from build123d import *

# Parameters (mm, degrees)
F1_DEPTH = 24
F3_DEPTH = 13


with BuildPart() as f1:
    # F0 (on Front) → F1 (new body)
    with BuildSketch(Plane.XZ):
        Polygon((30.517951, 0), (-33.758782, 0), (-56.984834, -93.20651), (58.065102, -93.20651), align=None)
    extrude(amount=F1_DEPTH)

    # F2 (on face) → F3 (join)
    with BuildSketch(Plane.XZ.offset(24)):
        Polygon((-51.863408, -72.654148), (-56.984834, -93.20651), (58.065102, -93.20651), (51.990858, -72.654148), align=None)
    extrude(amount=F3_DEPTH)


solid = f1.part
Part model, mm, in its own coordinate system. A direction names the side the tool comes from. Round coordinates to 2 decimals unless told otherwise and drop trailing zeros. Loops run counter-clockwise (first coordinate to the right, second up) from the corner with the lowest first, then second, coordinate; pieces in that order, holes last. Notation, with made-up numbers: (30.25, -20) - (48.25, -20) arc R8 ccw to (48.25, -14) - close; hole circle Ø4 at (-32, 18). An arc over 180 degrees is marked (long way). Answer as a JSON object with one key per item and string values.
Item 1: Band-saw the part on B-B on y = -34. List the corners of the cut face in (x, z).
Output:
{"outline": "(-56.98, -93.21) - (58.07, -93.21) - (51.99, -72.65) - (-51.86, -72.65) - close"}
Item 2: Band-saw the part on C-C on z = -77.5. List the corners of the cut face in (x, y).
Output:
{"outline": "(-53.07, -37) - (53.42, -37) - (53.42, 0) - (-53.07, 0) - close"}
Item 3: Pin check, flat tips, straight feed: pin 1 (4 mm diameter, centred on x = -33.5, z = -55.5, fed in from -Y); pin 2 (8 mm diameter, centred on y = -11.5, z = -69.5, fed in from +X); pin 3 (1 mm diameter, centred on y = -13.5, z = -61.5, fed in from -X). Stop position of each tip, or through.
Output:
{"pin 1": "y = -24", "pin 2": "x = 52.24", "pin 3": "x = -49.21"}
Item 4: Tool access for faces 1 (the face through (2, -24, -36)), 2 (the face through (0, -37, -83)): list every direction of +Z, -Z, +X, -X, +Y, -Y with a clear straight run to the whole face (end or side of a thin tool).
Output:
{"face 1": "+Z, +X, -X, -Y", "face 2": "+Z, -Z, +X, -X, -Y"}
Item 5: Wall check: L1, parallel to Z at x = -47, y = -33.5; L2, parallel to Y at x = 42.5, z = -68; L3, parallel to X at y = -6.5, z = -34.5. Give the ranges that are in metal, low to high.
Output:
{"L1": "-93.21 to -72.65", "L2": "-24 to 0", "L3": "-42.36 to 40.71"}
Item 6: Band-saw the part on D-D on x = 45. List the corners of the cut face in (y, z).
Output:
{"outline": "(-37, -93.21) - (0, -93.21) - (0, -49) - (-24, -49) - (-24, -72.65) - (-37, -72.65) - close"}
Item 7: Band-saw the part on A-A on x = -3. List the corners of the cut face in (y, z), plus the area to 3 significant figures.
Output:
{"outline": "(-37, -93.21) - (0, -93.21) - (0, 0) - (-24, 0) - (-24, -72.65) - (-37, -72.65) - close", "area": "2,500 mm2"}
